from build123d import *

# Parameters (mm, degrees)
CROQUIS1_W              = 18.9
CROQUIS1_H              = 9
SALIENTE_EXTRUIR1_DEPTH = 2
SALIENTE_EXTRUIR2_DEPTH = 3
CROQUIS3_R              = 1.6
SALIENTE_EXTRUIR4_DEPTH = 5


with BuildPart() as part:
    # Croquis1 → Saliente-Extruir1 (new body)
    with BuildSketch(Plane(origin=(0, 0, 0), x_dir=(1, 0, 0), z_dir=(0, 1, 0))):
        Polygon((23, 17), (-23, 17), (-23, 12.6), (0.3, 12.6), (0.3, 2), (-23, 2), (-23, -17), (23, -17), align=None)
        Polygon((12.3, 12.6), (18.6, 12.6), (18.6, 9), (20, 9), (20, -9), (18.6, -9), (18.6, -12.6), (12.3, -12.6), align=None, mode=Mode.SUBTRACT)
        with Locations((-9.15, -8.1)):
            Rectangle(CROQUIS1_W, CROQUIS1_H, mode=Mode.SUBTRACT)
    extrude(amount=-SALIENTE_EXTRUIR1_DEPTH)

    # Croquis2 → Saliente-Extruir2 (add)
    with BuildSketch(Plane.XZ.offset(2)):
        Polygon((-23, -17), (-23, -12.6), (-23, -2), (-23, 17), (23, 17), (23, -17), align=None)
        Polygon((-20, -14), (20, -14), (20, 14), (-20, 14), (-20, -2), (-20, -12.6), align=None, mode=Mode.SUBTRACT)
    extrude(amount=SALIENTE_EXTRUIR2_DEPTH)

    # Croquis3 → Saliente-Extruir4 (add, through all)
    # profile 1 of 6: a face of its own
    with BuildSketch(Plane(origin=(0, 0, 0), x_dir=(1, 0, 0), z_dir=(0, 1, 0))):
        Polygon((-16.07179677, -25), (-13.762395693, -21), (-16.07179677, -17), (-20.690598923, -17), (-23, -21), (-20.690598923, -25), align=None)
        with Locations(Location((-18.381197846, -21, 0), (0, 0, 270))):
            Circle(CROQUIS3_R, mode=Mode.SUBTRACT)
    # profile 2 of 6: a face of its own
    with BuildSketch(Plane(origin=(0, 0, 0), x_dir=(1, 0, 0), z_dir=(0, 1, 0))):
        Polygon((16.07179677, -25), (13.762395693, -21), (16.07179677, -17), (20.690598923, -17), (23, -21), (20.690598923, -25), align=None)
        with Locations(Location((18.381197846, -21, 0), (0, 0, 270))):
            Circle(CROQUIS3_R, mode=Mode.SUBTRACT)
    # profile 3 of 6: a face of its own
    with BuildSketch(Plane(origin=(0, 0, 0), x_dir=(1, 0, 0), z_dir=(0, 1, 0))):
        Polygon((-23, -17), (-20.690598923, -17), (-23, -21), align=None)
    # profile 4 of 6: a face of its own
    with BuildSketch(Plane(origin=(0, 0, 0), x_dir=(1, 0, 0), z_dir=(0, 1, 0))):
        Polygon((-13.762395693, -21), (-16.07179677, -17), (-13.762395693, -17), align=None)
    # profile 5 of 6: a face of its own
    with BuildSketch(Plane(origin=(0, 0, 0), x_dir=(1, 0, 0), z_dir=(0, 1, 0))):
        Polygon((13.762395693, -17), (16.07179677, -17), (13.762395693, -21), align=None)
    # profile 6 of 6: a face of its own
    with BuildSketch(Plane(origin=(0, 0, 0), x_dir=(1, 0, 0), z_dir=(0, 1, 0))):
        Polygon((20.690598923, -17), (23, -17), (23, -21), align=None)
    extrude(amount=-SALIENTE_EXTRUIR4_DEPTH)


solid = part.part
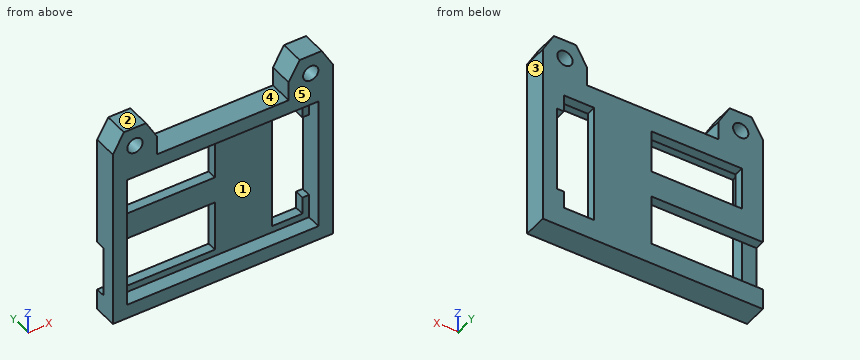
Model file for the job. Use its own axes, mm. Face numbers are marked on the shaded views. A direction names the side the tool comes from. Give positions to 0.01 mm unless a question says otherwise; leave off trailing zeros. Loops run counter-clockwise (first coordinate to the right, second up) from the corner with the lowest first, then second, coordinate; pieces in that order, holes last.
1) Wall check: line 1 (Z direction, x = -12.5, y = -1.3); line 2 (X direction, y = -2.15, z = 21); line 3 (X direction, y = -4.55, z = 5.5). Give the ranges that are in metal, low to high.
2) Pull direction X, two halves, no side cores. Call the marked faces 1, 2 and 3: +X half, -X half, draft (parallel to the pull), parting line (faces both ways), or undercut.
3) Saw through at C-C (z = 18.5). Write the cut outline in (x, y), plus the area to 3 significant figures.
4) Saw through at D-D (z = -11.5). Write the cut outline in (x, y), plus the area to 3 significant figures.
5) Tool access for the marked faces 4 and 5: list every direction of +Z, -Z, +X, -X, +Y, -Y with a clear straight run to the whole face (end or side of a thin tool).
6) Flat gauge pins, fed straight in: pin 1 Ø8.5 at (x, z) = (10, 6.5) entering from -Y; pin 2 Ø1.5 at (x, z) = (-21, -7.5) entering from +Y; pin 3 Ø2 at (x, y) = (15, -1) entering from +Z. Where does each tip first touch, or does it go through?
7) Saw through at A-A (z = 7). Write the cut outline in (x, y), plus the area to 3 significant figures.
8) Saw through at B-B (x = -13). Write the cut outline in (y, z).
Answer block:
1. line 1: z = -17 to -12.6, -2 to 3.6, 12.6 to 17
1. line 2: x = -23 to -19.98, -16.78 to -13.76, 13.76 to 16.78, 19.98 to 23
1. line 3: x = -23 to -20, 20 to 23
2. face 1: undercut
2. face 2: draft
2. face 3: +X half
3. outline: (-23, -5) - (-13.76, -5) - (-13.76, 0) - (-23, 0) - close; (13.76, -5) - (23, -5) - (23, 0) - (13.76, 0) - close
3. area: 92.4 mm2
4. outline: (-23, -5) - (-20, -5) - (-20, -2) - (-23, -2) - close; (0.3, -2) - (12.3, -2) - (12.3, 0) - (0.3, 0) - close; (18.6, -2) - (20, -2) - (20, -5) - (23, -5) - (23, 0) - (18.6, 0) - close
4. area: 50.8 mm2
5. face 4: +Z, +Y, -Y
5. face 5: +Z, -Z, +X, -X, -Y
6. pin 1: stops at y = -2
6. pin 2: stops at y = -2
6. pin 3: stops at z = 24.88
7. outline: (-23, -5) - (-20, -5) - (-20, -2) - (-18.6, -2) - (-18.6, 0) - (-23, 0) - close; (0.3, -2) - (12.3, -2) - (12.3, 0) - (0.3, 0) - close; (20, -5) - (23, -5) - (23, 0) - (20, 0) - close
7. area: 56.8 mm2
8. outline: (-5, -17) - (0, -17) - (0, -12.6) - (-2, -12.6) - (-2, -14) - (-5, -14) - close; (-5, 14) - (-2, 14) - (-2, 12.6) - (0, 12.6) - (0, 17) - (-5, 17) - close; (-2, -2) - (0, -2) - (0, 3.6) - (-2, 3.6) - close
